from build123d import *

# Parameters (mm, degrees)
EXTRUDE_1_DEPTH      = 9
SKETCH_2_W           = 9
SKETCH_2_H           = 9
EXTRUDE_2_DEPTH      = 2
EXTRUDE_5_DEPTH      = 9.5
EXTRUDE_5_DEPTH_BACK = 18.5
SKETCH_3_W           = 2
SKETCH_3_H           = 9
SKETCH_5_W           = 9
SKETCH_5_H           = 2
EXTRUDE_6_DEPTH      = 10
FILLET_2_R           = 2


with BuildPart() as part:
    # 草图1 → 凸台-拉伸1 (new body)
    with BuildSketch(Plane(origin=(0, 0, 0), x_dir=(1, 0, 0), z_dir=(0, 1, 0))):
        with BuildLine():
            ThreePointArc((15.854056032, 29.540059463), (0.854056032, 22.664455), (-14.145943968, 29.540059463))
            Line((-14.145943968, 29.540059463), (-14.145943968, -0.459940537))
            Line((-14.145943968, -0.459940537), (15.854056032, -0.459940537))
            Line((15.854056032, -0.459940537), (15.854056032, 29.540059463))
        make_face()
    extrude(amount=EXTRUDE_1_DEPTH)

    # 草图2 → 凸台-拉伸2 (add)
    with BuildSketch(Plane.ZY.offset(14.145943968)):
        with Locations((-4.040059463, 4.5)):
            Rectangle(SKETCH_2_W, SKETCH_2_H)
    extrude(amount=EXTRUDE_2_DEPTH)

    # 草图3 → 凸台-拉伸5 (add, two sides: drawn at the far end of the back side and taken through both)
    with BuildSketch(Plane(origin=(0, 9, 0), x_dir=(1, 0, 0), z_dir=(0, 1, 0)).offset(-EXTRUDE_5_DEPTH_BACK)):
        with Locations((-17.145943968, 4.040059463)):
            Rectangle(SKETCH_3_W, SKETCH_3_H)
    extrude(amount=EXTRUDE_5_DEPTH + EXTRUDE_5_DEPTH_BACK)

    # 草图5 → 凸台-拉伸6 (add)
    with BuildSketch(Plane.ZY.offset(18.145943968)):
        with Locations((-4.040059463, 17.5)):
            Rectangle(SKETCH_5_W, SKETCH_5_H)
        with Locations((-4.040059463, -8.5)):
            Rectangle(SKETCH_5_W, SKETCH_5_H)
    extrude(amount=EXTRUDE_6_DEPTH)

    # 圆角2
    fillet_2_edges = [part.edges().sort_by_distance(p)[0] for p in [
        (-16.145943968, 0, -4.040059463),
        (-16.145943968, 9, -4.040059463),
    ]]
    fillet(fillet_2_edges, radius=FILLET_2_R)


solid = part.part
The listing builds one solid part. Answer for the finished solid, in the listing's coordinates (mm). A direction names the side the tool comes from. Coordinates: 2 decimals unless noted, no trailing zeros. Write each loop counter-clockwise with the first axis right and the second up, starting at its lowest first coordinate (ties: lowest second). Pieces come first, ordered by that corner, then holes. Notation, with made-up numbers: M -32.75,-38 L 4.25,-38 A20 cw 4.25,-20 Z; hole C 10,-15.5 d1. An arc over 180 degrees is marked long. Put each result on its own line as item: value. Start each with the question number.
1. Consider line 1 (Y direction, x = -19.5, z = -5.5); line 2 (Z direction, x = -22.5, y = 17); line 3 (Y direction, x = 3, z = -16). Determine where each line is inside the solid, lowest interval first. Write a range as from..to.
2. Flat-ended cylindrical pins translate along their axes: P1, Ø2.5, axis at y = 3.5, z = -2.5, coming from the -X side; P2, Ø8, axis at y = 13.5, z = -2, coming from the +X side; P3, Ø4, axis at x = -20, y = -0.5, coming from the -Z side. Find the tip coordinate at first contact, or state that the pin passes through.
3. A cutting plane is placed at D-D on z = -25. Write down the section's boundary in (x, y), then the cut area to 3 significant figures.
4. Which of the six approach directions +Z, -Z, +X, -X, +Y, -Y give full straight-line access (tool end or side, diameter ignored) to faces 5 (the flat face through (1, 9, -11)), 6 (the flat face through (-18.146, 4, -4)), 7 (the flat face through (-16.146, -6, -4)), 8 (the flat face through (-17.9, 4.3, -8.54))?
5. A cutting plane is placed at B-B on z = -4. Write down the section's boundary in (x, y).
6. A cutting plane is placed at A-A on x = -19. Write down the section's boundary in (y, z).
7. For a pull along Y with two mould halves and no side action, classify faces 1 (the flat face through (-22, -9.5, -4)), 2 (the flat face through (-22, 18.5, -4)), 3 (the flat face through (-23, -7.5, -4)), 4 (the flat face through (-16.146, 15, -4)) as pulls with the +Y half, pulls with the -Y half, needs draft (parallel to the pull), parting line crosses it, or undercut.
8. A cutting plane is placed at C-C on y = 7.5. Write down the section's boundary in (x, z), then the cut area to 3 significant figures.
Resolved:
1. line 1: y = -9.5..-7.5, 16.5..18.5
1. line 2: z = -8.54..0.46
1. line 3: y = 0..9
2. P1: stops at x = -18.15
2. P2: stops at x = -15.47
2. P3: stops at z = -8.54
3. outline: M -14.15,0 L -8.48,0 L -8.48,9 L -14.15,9 Z; M 10.18,0 L 15.85,0 L 15.85,9 L 10.18,9 Z
3. area: 102 mm2
4. face 5: +Z, -Z, +X, +Y
4. face 6: +Z, -Z, -X
4. face 7: +Z, -Z, +X, -Y
4. face 8: -Z, -X, +Y, -Y
5. outline: M -28.15,-9.5 L -16.15,-9.5 L -16.15,-2 A2 cw -14.15,0 L 15.85,0 L 15.85,9 L -14.15,9 A2 cw -16.15,11 L -16.15,18.5 L -28.15,18.5 L -28.15,16.5 L -18.15,16.5 L -18.15,-7.5 L -28.15,-7.5 Z
6. outline: M -9.5,-8.54 L -7.5,-8.54 L -7.5,0.46 L -9.5,0.46 Z; M 16.5,-8.54 L 18.5,-8.54 L 18.5,0.46 L 16.5,0.46 Z
7. face 1: pulls with the -Y half
7. face 2: pulls with the +Y half
7. face 3: undercut
7. face 4: needs draft
8. outline: M -18.15,-8.54 L -14.15,-8.54 L -14.15,-29.54 A19.8 cw 15.85,-29.54 L 15.85,0.46 L -18.15,0.46 Z
8. area: 793 mm2
